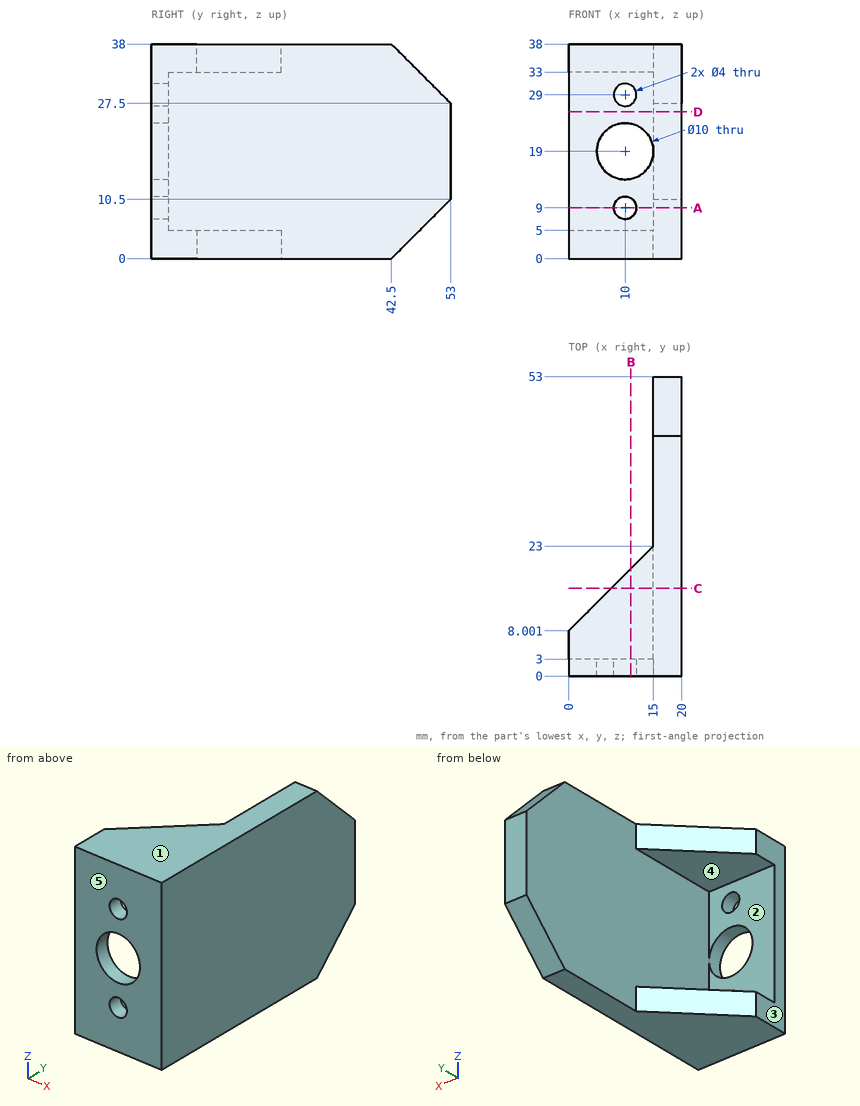
The figure shows three views and two pictorial views of one solid part (mm, origin at its lowest corner). Answer the questions. A direction names the side the tool comes from. Coordinates: 2 decimals unless noted, no trailing zeros. Order: outer loops, then holes, each group sorted by start corner. A loop starts at its lowest first (then second) coordinate and runs counter-clockwise, first axis right, second up.
Q1. A cutting plane is placed at D-D, the plane z = 26. Write down the section's boundary in (x, y), and give its area (3 significant figures).
Q2. A cutting plane is placed at B-B, the plane x = 11. Write down the section's boundary in (y, z), and give its area (3 significant figures).
Q3. A cutting plane is placed at C-C, the plane y = 15.5. Write down the section's boundary in (x, z), and give its area (3 significant figures).
Q4. Given P1, Ø3.5, axis at x = 10, z = 29, coming from the -Y side; P2, Ø12, axis at y = 9.5, z = 17, coming from the -X side; P3, Ø1.5, axis at x = 10.5, z = 4.5, coming from the +Y side; P4, Ø5, axis at x = 10, z = 9, coming from the +Y side, each flat-ended and moving along its own axis, determine where each tip first touches the part or whether it passes through.
Q5. Consider line 1 (Z direction, x = 10, y = 0.75); line 2 (X direction, y = 0.85, z = 9); line 3 (X direction, y = 0.95, z = 19). Determine where each line is inside the solid, lowest interval first.
Q6. For a pull along Z with two mould halves and no side action, classify the marked faces 1, 2 and 3 as pulls with the +Z half, pulls with the -Z half, needs draft (parallel to the pull), parting line crosses it, or undercut.
Q7. Which of the six approach directions +Z, -Z, +X, -X, +Y, -Y give full straight-line access (tool end or side, diameter ignored) to the marked faces 4 and 5?
Q8. A cutting plane is placed at A-A, the plane z = 9. Write down the section's boundary in (x, y).
Answers follow:
1. outline: (0, 0) - (20, 0) - (20, 53) - (15, 53) - (15, 3) - (0, 3) - close
1. area: 310 mm2
2. outline: (0, 0) - (19, 0) - (19, 5) - (3, 5) - (3, 7.27) - (0, 7.27) - close; (0, 10.73) - (3, 10.73) - (3, 14.1) - (0, 14.1) - close; (0, 23.9) - (3, 23.9) - (3, 27.27) - (0, 27.27) - close; (0, 30.73) - (3, 30.73) - (3, 33) - (19, 33) - (19, 38) - (0, 38) - close
2. area: 224 mm2
3. outline: (7.5, 0) - (20, 0) - (20, 38) - (7.5, 38) - (7.5, 33) - (15, 33) - (15, 5) - (7.5, 5) - close
3. area: 265 mm2
4. P1: passes through
4. P2: stops at x = 15
4. P3: stops at y = 19.25
4. P4: stops at y = 3
5. line 1: z = 0 to 7, 11 to 14, 24 to 27, 31 to 38
5. line 2: x = 0 to 8, 12 to 20
5. line 3: x = 0 to 5, 15 to 20
6. face 1: pulls with the +Z half
6. face 2: undercut
6. face 3: needs draft
7. face 4: -X, +Y
7. face 5: +Z, -Z, +X, -X, -Y
8. outline: (0, 0) - (8, 0) - (8, 3) - (0, 3) - close; (12, 0) - (20, 0) - (20, 51.5) - (15, 51.5) - (15, 3) - (12, 3) - close
